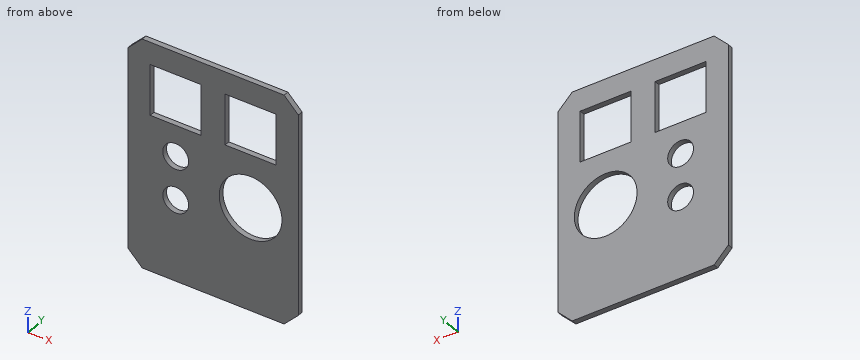
```python
from build123d import *

# Parameters (mm, degrees)
F0_W     = 151.638
F0_H     = 204
F0_R     = 11.5
F0_R_2   = 27.94
F0_W_2   = 45.339
F0_H_2   = 45.339
F1_DEPTH = 4.7625
F2_SIZE  = 12.7


with BuildPart() as f1:
    # F0 (on Front) → F1 (new body)
    with BuildSketch(Plane.XZ):
        with Locations((75.819, -102)):
            Rectangle(F0_W, F0_H)
        with Locations((42.502667, -131.689877)):
            Circle(F0_R, mode=Mode.SUBTRACT)
        with Locations((109.135333, -112.280877)):
            Circle(F0_R_2, mode=Mode.SUBTRACT)
        with Locations((42.502667, -92.871877)):
            Circle(F0_R, mode=Mode.SUBTRACT)
        with Locations((42.502667, -42.502667)):
            Rectangle(F0_W_2, F0_H_2, mode=Mode.SUBTRACT)
        with Locations((109.135333, -42.502667)):
            Rectangle(F0_W_2, F0_H_2, mode=Mode.SUBTRACT)
    extrude(amount=F1_DEPTH)

    # F2
    f2_edges = [f1.edges().sort_by_distance(p)[0] for p in [
        (151.638, -2.38125, 0),
        (0, -2.38125, 0),
        (0, -2.38125, -204),
        (151.638, -2.38125, -204),
    ]]
    chamfer(f2_edges, length=F2_SIZE)


solid = f1.part
```
Geometry check sheet. Reference: the model listing, model coordinates, mm. Give positions to 0.01 mm unless a question says otherwise; leave off trailing zeros. Order: outer loops, then holes, each group sorted by start corner. A loop starts at its lowest first (then second) coordinate and runs counter-clockwise, first axis right, second up. Notation, with made-up numbers: (66, 22) -> (79, 22) arc R9 ccw to (79, 30) -> close; hole circle Ø1 at (-28.5, 20). An arc over 180 degrees is marked (long way). Write each question's results on one line, items separated by ' | '. Start each with the question number.
(1) Sectioned sample at D-D (y = -3.35). Enter the section's corners in (x, z).
(2) Sectioned sample at B-B (z = -42). Enter the section's corners in (x, y).
(3) Scan lines: line 1 (X direction, y = -2.15, z = -61.5); line 2 (Z direction, x = 101.5, y = -0.8); line 3 (Z direction, x = 59.5, y = -2.15). Record each from-to range of solid material in increasing order.
(4) Sectioned sample at A-A (x = 24.5). Enter the section's corners in (y, z), plus the area to 3 significant figures.
(5) Sectioned sample at C-C (x = 118.5). Enter the section's corners in (y, z), plus the area to 3 significant figures.
Answer below:
1) outline: (0, -191.3) -> (12.7, -204) -> (138.94, -204) -> (151.64, -191.3) -> (151.64, -12.7) -> (138.94, 0) -> (12.7, 0) -> (0, -12.7) -> close; hole (19.83, -65.17) -> (65.17, -65.17) -> (65.17, -19.83) -> (19.83, -19.83) -> close; hole circle Ø23 at (42.5, -131.69); hole circle Ø23 at (42.5, -92.87); hole circle Ø55.88 at (109.14, -112.28); hole (86.47, -65.17) -> (131.8, -65.17) -> (131.8, -19.83) -> (86.47, -19.83) -> close
2) outline: (0, -4.76) -> (19.83, -4.76) -> (19.83, 0) -> (0, 0) -> close; (65.17, -4.76) -> (86.47, -4.76) -> (86.47, 0) -> (65.17, 0) -> close; (131.8, -4.76) -> (151.64, -4.76) -> (151.64, 0) -> (131.8, 0) -> close
3) line 1: 0 to 19.83, 65.17 to 86.47, 131.8 to 151.64 | line 2: -204 to -139.16, -85.4 to -65.17, -19.83 to 0 | line 3: -204 to -65.17, -19.83 to 0
4) outline: (-4.76, -204) -> (0, -204) -> (0, -65.17) -> (-4.76, -65.17) -> close; (-4.76, -19.83) -> (0, -19.83) -> (0, 0) -> (-4.76, 0) -> close | area: 756 mm2
5) outline: (-4.76, -204) -> (0, -204) -> (0, -138.6) -> (-4.76, -138.6) -> close; (-4.76, -85.96) -> (0, -85.96) -> (0, -65.17) -> (-4.76, -65.17) -> close; (-4.76, -19.83) -> (0, -19.83) -> (0, 0) -> (-4.76, 0) -> close | area: 505 mm2
